Part model, mm, in its own coordinate system. A direction names the side the tool comes from. Give positions to 0.01 mm unless a question says otherwise; leave off trailing zeros. Order: outer loops, then holes, each group sorted by start corner. A loop starts at its lowest first (then second) coordinate and runs counter-clockwise, first axis right, second up. Notation, with made-up numbers: (0.5, 85) - (22.5, 85) arc R10 ccw to (22.5, 97) - close; hole circle Ø10 at (-28, -31). An arc over 180 degrees is marked (long way). One line per item, written item: value.
```python
from build123d import *

# Parameters (mm, degrees)
SKETCH1_W           = 78.74
SKETCH1_H           = 34.29
BOSS_EXTRUDE1_DEPTH = 1.5875
CUT_EXTRUDE1_REACH  = 87.897
SKETCH2_R           = 1.5875
SKETCH3_W           = 5.588
SKETCH3_H           = 10.16
SKETCH3_H_2         = 17.78
SKETCH3_H_3         = 12.7
BOSS_EXTRUDE2_DEPTH = 7.112
SKETCH4_W           = 6.35
SKETCH4_H           = 6.35
BOSS_EXTRUDE3_DEPTH = 3.81
BOSS_EXTRUDE4_DEPTH = 4.0005
SKETCH6_W           = 1.27
SKETCH6_H           = 3.048
BOSS_EXTRUDE5_DEPTH = 1.27


with BuildPart() as part:
    # Sketch1 → Boss-Extrude1 (new body)
    with BuildSketch(Plane.XY):
        with Locations((39.37, 17.145)):
            Rectangle(SKETCH1_W, SKETCH1_H)
    extrude(amount=BOSS_EXTRUDE1_DEPTH)

    # Sketch2 → Cut-Extrude1 (cut, up to next)
    with BuildSketch(Plane.XY.offset(1.5875), mode=Mode.PRIVATE) as cut_extrude1_sk1:
        with Locations((2.921, 3.429)):
            Circle(SKETCH2_R)
    cut_extrude1_tool1 = extrude(cut_extrude1_sk1.sketch, amount=-CUT_EXTRUDE1_REACH, mode=Mode.PRIVATE) & part.part
    # Sketch2 → Cut-Extrude1 (cut, up to next)
    with BuildSketch(Plane.XY.offset(1.5875), mode=Mode.PRIVATE) as cut_extrude1_sk2:
        with Locations((2.921, 24.4856)):
            Circle(SKETCH2_R)
    cut_extrude1_tool2 = extrude(cut_extrude1_sk2.sketch, amount=-CUT_EXTRUDE1_REACH, mode=Mode.PRIVATE) & part.part
    # Sketch2 → Cut-Extrude1 (cut, up to next)
    with BuildSketch(Plane.XY.offset(1.5875), mode=Mode.PRIVATE) as cut_extrude1_sk3:
        with Locations((46.609, 24.4856)):
            Circle(SKETCH2_R)
    cut_extrude1_tool3 = extrude(cut_extrude1_sk3.sketch, amount=-CUT_EXTRUDE1_REACH, mode=Mode.PRIVATE) & part.part
    # Sketch2 → Cut-Extrude1 (cut, up to next)
    with BuildSketch(Plane.XY.offset(1.5875), mode=Mode.PRIVATE) as cut_extrude1_sk4:
        with Locations((46.609, 3.429)):
            Circle(SKETCH2_R)
    cut_extrude1_tool4 = extrude(cut_extrude1_sk4.sketch, amount=-CUT_EXTRUDE1_REACH, mode=Mode.PRIVATE) & part.part
    add(cut_extrude1_tool1.solids().sort_by_distance((2.921, 3.429, 1.5875))[0], mode=Mode.SUBTRACT)
    add(cut_extrude1_tool2.solids().sort_by_distance((2.921, 24.4856, 1.5875))[0], mode=Mode.SUBTRACT)
    add(cut_extrude1_tool3.solids().sort_by_distance((46.609, 24.4856, 1.5875))[0], mode=Mode.SUBTRACT)
    add(cut_extrude1_tool4.solids().sort_by_distance((46.609, 3.429, 1.5875))[0], mode=Mode.SUBTRACT)

    # Sketch3 → Boss-Extrude2 (add)
    with BuildSketch(Plane.XY.offset(1.5875)):
        with Locations((54.102, 27.94)):
            Rectangle(SKETCH3_W, SKETCH3_H)
        with Locations((60.96, 24.13)):
            Rectangle(SKETCH3_W, SKETCH3_H_2)
        with Locations((67.818, 24.13)):
            Rectangle(SKETCH3_W, SKETCH3_H_2)
        with Locations((74.676, 24.13)):
            Rectangle(SKETCH3_W, SKETCH3_H_2)
        with Locations((60.96, 8.89)):
            Rectangle(SKETCH3_W, SKETCH3_H)
        with Locations((67.818, 8.89)):
            Rectangle(SKETCH3_W, SKETCH3_H)
        with Locations((74.676, 7.62)):
            Rectangle(SKETCH3_W, SKETCH3_H_3)
    extrude(amount=BOSS_EXTRUDE2_DEPTH)

    # Sketch4 → Boss-Extrude3 (add)
    with BuildSketch(Plane.XY.offset(1.5875)):
        with Locations((53.721, 7.366)):
            Rectangle(SKETCH4_W, SKETCH4_H)
    extrude(amount=BOSS_EXTRUDE3_DEPTH)

    # Sketch5 → Boss-Extrude4 (add, symmetric)
    with BuildSketch(Plane(origin=(0, 15.875, 0), x_dir=(-1, 0, 0), z_dir=(0, -1, 0))):
        Polygon((-24.13, 9.525), (-19.177, 9.525), (-19.177, 0), (-17.907, 0), (-17.907, 8.128), (-7.493, 8.128), (-7.493, 0), (-6.223, 0), (-6.223, 9.525), (-1.27, 9.525), (-1.27, 10.16), (-6.858, 10.16), (-6.858, 8.763), (-18.542, 8.763), (-18.542, 10.16), (-24.13, 10.16), align=None)
    extrude(amount=BOSS_EXTRUDE4_DEPTH, both=True)

    # Sketch6 → Boss-Extrude5 (add)
    with BuildSketch(Plane.XY.offset(1.5875)):
        with Locations((37.465, 31.496)):
            Rectangle(SKETCH6_W, SKETCH6_H)
        with Locations((31.115, 31.496)):
            Rectangle(SKETCH6_W, SKETCH6_H)
        with Locations((24.765, 31.496)):
            Rectangle(SKETCH6_W, SKETCH6_H)
        with Locations((18.415, 31.496)):
            Rectangle(SKETCH6_W, SKETCH6_H)
    extrude(amount=BOSS_EXTRUDE5_DEPTH)


solid = part.part
```
1) Cut at D-D, the plane x = 74.5. Give the cut face in (y, z).
Outcome:
outline: (0, 0) - (34.29, 0) - (34.29, 1.59) - (33.02, 1.59) - (33.02, 8.7) - (15.24, 8.7) - (15.24, 1.59) - (13.97, 1.59) - (13.97, 8.7) - (1.27, 8.7) - (1.27, 1.59) - (0, 1.59) - close
2) Drill centre lines: line 1 along X through (y, z) = (25.5, 3.25); line 2 along X through (y, z) = (19, 4); line 3 along X through (y, z) = (7.5, 2.5). Where is each one in solid material? Low to high. Write a range as from..to.
Outcome:
line 1: x = 51.31..56.9, 58.17..63.75, 65.02..70.61, 71.88..77.47
line 2: x = 58.17..63.75, 65.02..70.61, 71.88..77.47
line 3: x = 50.55..56.9, 58.17..63.75, 65.02..70.61, 71.88..77.47
3) Which spindle directions (+Z, -Z, +X, -X, +Y, -Y) get a long thin tool onto all of the face, cutting with end or side? Do faces 4 (the flat face through (4, 16, -9.525)), 5 (the flat face through (61, 13.97, 5)), 6 (the flat face through (75, 8, 8.7)), 7 (the flat face through (77.47, 24, 5)), 8 (the flat face through (65.024, 24, 5)). Say none if no direction does.
Outcome:
face 4: -X, +Y, -Y
face 5: +Z, +X, -X
face 6: +Z, +X, -X, +Y, -Y
face 7: +Z, +X, +Y, -Y
face 8: +Z, +Y, -Y
4) Cut at C-C, the plane y = 6.5. Give the cut face in (x, z).
Outcome:
outline: (0, 0) - (78.74, 0) - (78.74, 1.59) - (77.47, 1.59) - (77.47, 8.7) - (71.88, 8.7) - (71.88, 1.59) - (70.61, 1.59) - (70.61, 8.7) - (65.02, 8.7) - (65.02, 1.59) - (63.75, 1.59) - (63.75, 8.7) - (58.17, 8.7) - (58.17, 1.59) - (56.9, 1.59) - (56.9, 5.4) - (50.55, 5.4) - (50.55, 1.59) - (0, 1.59) - close
5) Pin check, flat tips, straight feed: pin 1 (2 mm diameter, centred on x = 58.5, z = 5, fed in from +Y); pin 2 (0.6 mm diameter, centred on x = 37.5, y = 32, fed in from +Z); pin 3 (1.1 mm diameter, centred on y = 14, z = -9.5, fed in from -X); pin 4 (3 mm diameter, centred on x = 46.61, y = 24.49, fed in from -Z). Stop position of each tip, or through.
Outcome:
pin 1: stops at y = 33.02
pin 2: stops at z = 2.86
pin 3: stops at x = 1.27
pin 4: passes through
6) Mould opens along Y. For faces 1 (the flat face through (78.74, 17, 1)), 2 (the flat face through (68, 3.81, 5)), 3 (the flat face through (68, 13.97, 5)) say: released by +Y, released by -Y, zero draft, split by the parting line, or undercut.
Outcome:
face 1: zero draft
face 2: released by -Y
face 3: undercut
7) Cut at B-B, the plane z = -4.5. Give the cut face in (x, y), then the cut area to 3 significant figures.
Outcome:
outline: (6.22, 11.87) - (7.49, 11.87) - (7.49, 19.88) - (6.22, 19.88) - close; (17.91, 11.87) - (19.18, 11.87) - (19.18, 19.88) - (17.91, 19.88) - close
area: 20.3 mm^2
